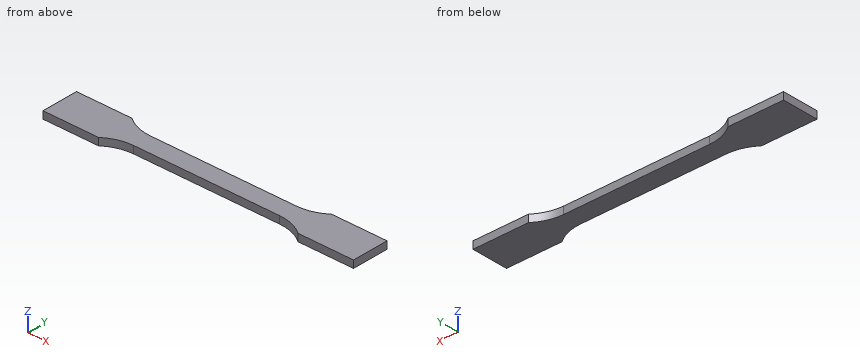
from build123d import *

# Parameters (mm, degrees)
BOSS_EXTRUDE1_DEPTH = 2


with BuildPart() as part:
    # Sketch1 → Boss-Extrude1 (new body, symmetric)
    with BuildSketch(Plane.XY):
        with BuildLine():
            Line((-85, 10), (-85, -10))
            Line((-85, -10), (-54.662878299, -10))
            ThreePointArc((-54.662878299, -10), (-47.745966692, -6.284366617), (-40, -5))
            Line((-40, -5), (40, -5))
            ThreePointArc((40, -5), (47.745966692, -6.284366617), (54.662878299, -10))
            Line((54.662878299, -10), (85, -10))
            Line((85, -10), (85, 10))
            Line((85, 10), (54.662878299, 10))
            ThreePointArc((54.662878299, 10), (47.745966692, 6.284366617), (40, 5))
            Line((40, 5), (-40, 5))
            ThreePointArc((-40, 5), (-47.745966692, 6.284366617), (-54.662878299, 10))
            Line((-54.662878299, 10), (-85, 10))
        make_face()
    extrude(amount=BOSS_EXTRUDE1_DEPTH, both=True)


solid = part.part
Design review of the part built by this model. Coordinates are the model's own, in mm. Coordinates: 2 decimals unless noted, no trailing zeros. Order: outer loops, then holes, each group sorted by start corner. A loop starts at its lowest first (then second) coordinate and runs counter-clockwise, first axis right, second up. Notation, with made-up numbers: M 16.25,81.25 L 37.25,81.25 A19 cw 37.25,86.25 Z; hole C 18,56 d7. An arc over 180 degrees is marked long. Use a Markdown table: item, result.
(1) Add section A-A (y = 7.75). Give the boundary of the cut face in (x, z), then the cut area to 3 significant figures.
Worked answers:
| item | result |
|---|---|
| outline | M -85,-2 L -51.16,-2 L -51.16,2 L -85,2 Z; M 51.16,-2 L 85,-2 L 85,2 L 51.16,2 Z |
| area | 271 mm2 |
(2) Add section B-B (z = -0.15). Give the boundary of the cut face in (x, y), then the cut area to 3 significant figures.
Worked answers:
| item | result |
|---|---|
| outline | M -85,-10 L -54.66,-10 A24 cw -40,-5 L 40,-5 A24 cw 54.66,-10 L 85,-10 L 85,10 L 54.66,10 A24 cw 40,5 L -40,5 A24 cw -54.66,10 L -85,10 Z |
| area | 2,400 mm2 |
(3) For P1, Ø2, axis at x = 42, z = 0.5, coming from the +Y side; P2, Ø1.2, axis at x = -18, z = 0, coming from the +Y side; P3, Ø1.5, axis at x = 12.5, z = -0.5, coming from the -Y side, all flat-tipped, find the tip position at first contact; note any pin that passes through.
Worked answers:
| item | result |
|---|---|
| P1 | stops at y = 5.19 |
| P2 | stops at y = 5 |
| P3 | stops at y = -5 |
(4) Add section C-C (x = -23.5). Give the boundary of the cut face in (y, z).
Worked answers:
| item | result |
|---|---|
| outline | M -5,-2 L 5,-2 L 5,2 L -5,2 Z |
(5) Wall thickness on probe 1 along Y at (x, z) = (-6.5, -1.35); probe 2 along X at (y, z) = (7, 0.65); probe 3 along Y at (x, z) = (-51.5, 1.35): over which ranges is each line inside the solid? List them lowest first.
Worked answers:
| item | result |
|---|---|
| probe 1 | y = -5 to 5 |
| probe 2 | x = -85 to -49.59, 49.59 to 85 |
| probe 3 | y = -7.93 to 7.93 |
(6) Add section D-D (x = -45). Give the boundary of the cut face in (y, z).
Worked answers:
| item | result |
|---|---|
| outline | M -5.53,-2 L 5.53,-2 L 5.53,2 L -5.53,2 Z |
